For this review, take the finished solid that the model builds, in its own axes (mm). Round coordinates to 2 decimals unless told otherwise and drop trailing zeros. Loops run counter-clockwise (first coordinate to the right, second up) from the corner with the lowest first, then second, coordinate; pieces in that order, holes last. Notation, with made-up numbers: M 52.25,-29.5 L 105.25,-29.5 A18 cw 105.25,-12.5 Z; hole C -10.5,37 d7. An arc over 180 degrees is marked long. Write item = value, one per line. Start each with the question number.
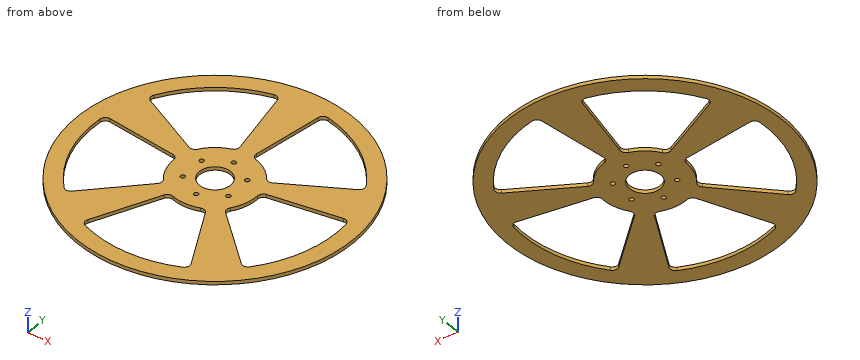
```python
from build123d import *

# Parameters (mm, degrees)
SKETCH1_R           = 127
SKETCH1_R_2         = 14.2875
SKETCH1_R_3         = 2.032
BOSS_EXTRUDE2_DEPTH = 3.175
FILLET1_R           = 5.08
FILLET3_R           = 5.08


with BuildPart() as part:
    # Sketch1 → Boss-Extrude2 (new body)
    with BuildSketch(Plane.XY):
        Circle(SKETCH1_R)
        Circle(SKETCH1_R_2, mode=Mode.SUBTRACT)
        with Locations((0, 23.876)):
            Circle(SKETCH1_R_3, mode=Mode.SUBTRACT)
        with Locations((20.677222541, 11.938)):
            Circle(SKETCH1_R_3, mode=Mode.SUBTRACT)
        with Locations((20.677222541, -11.938)):
            Circle(SKETCH1_R_3, mode=Mode.SUBTRACT)
        with Locations((0, -23.876)):
            Circle(SKETCH1_R_3, mode=Mode.SUBTRACT)
        with Locations((-20.677222541, -11.938)):
            Circle(SKETCH1_R_3, mode=Mode.SUBTRACT)
        with Locations((-20.677222541, 11.938)):
            Circle(SKETCH1_R_3, mode=Mode.SUBTRACT)
        with BuildLine():
            Line((19.448595899, 110.298468337), (6.615995569, 37.52117539))
            ThreePointArc((6.615995569, 37.52117539), (22.394618112, 30.823547486), (33.640303288, 17.886866542))
            Line((33.640303288, 17.886866542), (98.8901304, 52.580815032))
            ThreePointArc((98.8901304, 52.580815032), (65.831948257, 90.60990337), (19.448595899, 110.298468337))
        make_face(mode=Mode.SUBTRACT)
        with BuildLine():
            Line((-6.615995569, 37.52117539), (-19.448595899, 110.298468337))
            ThreePointArc((-19.448595899, 110.298468337), (-65.831948257, 90.60990337), (-98.8901304, 52.580815032))
            Line((-98.8901304, 52.580815032), (-33.640303288, 17.886866542))
            ThreePointArc((-33.640303288, 17.886866542), (-22.394618112, 30.823547486), (-6.615995569, 37.52117539))
        make_face(mode=Mode.SUBTRACT)
        with BuildLine():
            Line((37.729213419, 5.302495147), (110.910023699, 15.587387308))
            ThreePointArc((110.910023699, 15.587387308), (106.518329825, -34.60990337), (80.566057638, -77.801737491))
            Line((80.566057638, -77.801737491), (27.406846393, -26.466483914))
            ThreePointArc((27.406846393, -26.466483914), (36.235253271, -11.773547486), (37.729213419, 5.302495147))
        make_face(mode=Mode.SUBTRACT)
        with BuildLine():
            Line((49.09756844, -100.664933186), (16.701940693, -34.244053164))
            ThreePointArc((16.701940693, -34.244053164), (0, -38.1), (-16.701940693, -34.244053164))
            Line((-16.701940693, -34.244053164), (-49.09756844, -100.664933186))
            ThreePointArc((-49.09756844, -100.664933186), (0, -112), (49.09756844, -100.664933186))
        make_face(mode=Mode.SUBTRACT)
        with BuildLine():
            Line((-80.566057638, -77.801737491), (-27.406846393, -26.466483914))
            ThreePointArc((-27.406846393, -26.466483914), (-36.235253271, -11.773547486), (-37.729213419, 5.302495147))
            Line((-37.729213419, 5.302495147), (-110.910023699, 15.587387308))
            ThreePointArc((-110.910023699, 15.587387308), (-106.518329825, -34.60990337), (-80.566057638, -77.801737491))
        make_face(mode=Mode.SUBTRACT)
    extrude(amount=BOSS_EXTRUDE2_DEPTH)

    # Fillet1
    fillet1_edges = [part.edges().sort_by_distance(p)[0] for p in [
        (98.8901304, 52.580815032, 1.5875),
        (19.448595899, 110.298468337, 1.5875),
        (6.615995569, 37.52117539, 1.5875),
        (33.640303288, 17.886866542, 1.5875),
    ]]
    fillet(fillet1_edges, radius=FILLET1_R)

    # Fillet3
    fillet3_edges = [part.edges().sort_by_distance(p)[0] for p in [
        (-33.640303288, 17.886866542, 1.5875),
        (-6.615995569, 37.52117539, 1.5875),
        (-19.448595899, 110.298468337, 1.5875),
        (-98.8901304, 52.580815032, 1.5875),
        (37.729213419, 5.302495147, 1.5875),
        (27.406846393, -26.466483914, 1.5875),
        (80.566057638, -77.801737491, 1.5875),
        (110.910023699, 15.587387308, 1.5875),
        (-49.09756844, -100.664933186, 1.5875),
        (49.09756844, -100.664933186, 1.5875),
        (16.701940693, -34.244053164, 1.5875),
        (-16.701940693, -34.244053164, 1.5875),
        (-110.910023699, 15.587387308, 1.5875),
        (-80.566057638, -77.801737491, 1.5875),
        (-27.406846393, -26.466483914, 1.5875),
        (-37.729213419, 5.302495147, 1.5875),
    ]]
    fillet(fillet3_edges, radius=FILLET3_R)


solid = part.part
```
(1) Wall thickness on L1, parallel to Y at x = -1, z = 1.7; L2, parallel to X at y = 27.5, z = 2.6; L3, parallel to X at y = -61.5, z = 2.05: over which ranges is each line inside the solid? List them lowest first.
(2) Add section B-B on y = 92.5. Write out the cut boundary in (x, z) (3 decimals).
(3) For pin 1 Ø1 at (y, z) = (48, 1.5) entering from -X; pin 2 Ø1 at (y, z) = (-61, 2) entering from +X; pin 3 Ø1.5 at (y, z) = (-18, 1) entering from +X, all flat-tipped, find the tip position at first contact; note any pin that passes through.
(4) Add section A-A on x = 54.5. Write out the cut boundary in (y, z) (3 decimals), and give its area (3 significant figures).
(5) Add section C-C on x = -101.5. Write out the cut boundary in (y, z) (3 decimals).
(6) Add section D-D on z = 2.55. Count the separate pieces of the cut face and the enclosed holes in it, and give its area (3 significant figures).
Answer sheet:
q1.L1 = -127 to -112, -38.09 to -25.64, -22.11 to -14.25, 14.25 to 22.11, 25.64 to 127
q1.L2 = -123.99 to -51.72, -26.37 to 26.37, 51.72 to 123.99
q1.L3 = -111.12 to -93.6, -63.69 to -30, 30 to 63.69, 93.6 to 111.12
q2.outline = M -87.022,0 L -63.149,0 L -63.149,3.175 L -87.022,3.175 Z; M -16.31,0 L 16.31,0 L 16.31,3.175 L -16.31,3.175 Z; M 63.149,0 L 87.022,0 L 87.022,3.175 L 63.149,3.175 Z
q3.pin_1 = -117.78
q3.pin_2 = 111.66
q3.pin_3 = 125.82
q4.outline = M -114.712,0 L -52.63,0 L -52.63,3.175 L -114.712,3.175 Z; M 7.659,0 L 28.978,0 L 28.978,3.175 L 7.659,3.175 Z; M 97.846,0 L 114.712,0 L 114.712,3.175 L 97.846,3.175 Z
q4.area = 318 mm²
q5.outline = M -76.333,0 L -47.347,0 L -47.347,3.175 L -76.333,3.175 Z; M 14.265,0 L 76.333,0 L 76.333,3.175 L 14.265,3.175 Z
q6.separate_pieces = 1
q6.enclosed_holes = 12
q6.area = 24,900 mm²
